```python
from build123d import *

# Parameters (mm, degrees)
SKETCH1_R                                  = 55
SKETCH1_R_2                                = 5
BOSS_EXTRUDE1_DEPTH                        = 11
SKETCH2_R                                  = 7.5
CUT_EXTRUDE1_DEPTH                         = 1
SKETCH3_R                                  = 7
CUT_EXTRUDE2_DEPTH                         = 4
MIRROR1_AT_THE_SECOND_PLANE_COPY_1_SKETC_R = 7.5
MIRROR1_AT_THE_SECOND_PLANE_COPY_1_DEPTH   = 1
MIRROR1_AT_THE_SECOND_PLANE_COPY_2_SKETC_R = 7
MIRROR1_AT_THE_SECOND_PLANE_COPY_2_DEPTH   = 4
FILLET1_R                                  = 200


with BuildPart() as part:
    # Sketch1 → Boss-Extrude1 (new, symmetric)
    with BuildSketch(Plane(origin=(0, 0, 0), x_dir=(0, 0, -1), z_dir=(1, 0, 0))):
        with BuildLine():
            Line((-62.214626272, 32.083333333), (-13.33170563, 126.875))
            ThreePointArc((-13.33170563, 126.875), (0, 135), (13.33170563, 126.875))
            Line((13.33170563, 126.875), (51.962948302, 51.962948302))
            Line((51.962948302, 51.962948302), (126.875, 13.33170563))
            ThreePointArc((126.875, 13.33170563), (135, 0), (126.875, -13.33170563))
            Line((126.875, -13.33170563), (32.083333333, -62.214626272))
            ThreePointArc((32.083333333, -62.214626272), (-49.497474683, -49.497474683), (-62.214626272, 32.083333333))
        make_face()
        Circle(SKETCH1_R, mode=Mode.SUBTRACT)
        with Locations((0, 120)):
            Circle(SKETCH1_R_2, mode=Mode.SUBTRACT)
        with Locations(Location((120, 0, 0), (0, 0, 180))):
            Circle(SKETCH1_R_2, mode=Mode.SUBTRACT)
    extrude(amount=BOSS_EXTRUDE1_DEPTH, both=True)

    # Sketch2 → Cut-Extrude1 (cut)
    with BuildSketch(Plane(origin=(11, 0, 0), x_dir=(0, 0, -1), z_dir=(1, 0, 0))):
        with Locations((0, 120)):
            Circle(SKETCH2_R)
    cut_extrude1 = extrude(amount=-CUT_EXTRUDE1_DEPTH, mode=Mode.SUBTRACT)

    # Sketch3 → Cut-Extrude2 (cut)
    with BuildSketch(Plane(origin=(10, 0, 0), x_dir=(0, 0, -1), z_dir=(1, 0, 0))):
        with Locations((0, 120)):
            Circle(SKETCH3_R)
    cut_extrude2 = extrude(amount=-CUT_EXTRUDE2_DEPTH, mode=Mode.SUBTRACT)

    # Mirror1: Cut-Extrude1, Cut-Extrude2 across plane
    add(cut_extrude1.mirror(Plane(origin=(0, 0, 0), x_dir=(0, -0.7071067811865464, 0.7071067811865487), z_dir=(0, -0.7071067811865487, -0.7071067811865464))), mode=Mode.SUBTRACT)
    add(cut_extrude2.mirror(Plane(origin=(0, 0, 0), x_dir=(0, -0.7071067811865464, 0.7071067811865487), z_dir=(0, -0.7071067811865487, -0.7071067811865464))), mode=Mode.SUBTRACT)

    # Mirror1 at the second plane: Cut-Extrude1, Cut-Extrude2 across plane
    add(cut_extrude1.mirror(Plane(origin=(0, 0, 0), x_dir=(0, 0, 1), z_dir=(1, 0, 0))), mode=Mode.SUBTRACT)
    add(cut_extrude2.mirror(Plane(origin=(0, 0, 0), x_dir=(0, 0, 1), z_dir=(1, 0, 0))), mode=Mode.SUBTRACT)

    # Mirror1 at the second plane copy 1 sketc → Mirror1 at the second plane copy 1 (cut)
    with BuildSketch(Plane(origin=(-11, 0, 0), x_dir=(0, 1, 0), z_dir=(-1, 0, 0))):
        with Locations((0, 120)):
            Circle(MIRROR1_AT_THE_SECOND_PLANE_COPY_1_SKETC_R)
    extrude(amount=-MIRROR1_AT_THE_SECOND_PLANE_COPY_1_DEPTH, mode=Mode.SUBTRACT)

    # Mirror1 at the second plane copy 2 sketc → Mirror1 at the second plane copy 2 (cut)
    with BuildSketch(Plane(origin=(-10, 0, 0), x_dir=(0, 1, 0), z_dir=(-1, 0, 0))):
        with Locations((0, 120)):
            Circle(MIRROR1_AT_THE_SECOND_PLANE_COPY_2_SKETC_R)
    extrude(amount=-MIRROR1_AT_THE_SECOND_PLANE_COPY_2_DEPTH, mode=Mode.SUBTRACT)

    # Fillet1
    fillet1_edges = [part.edges().sort_by_distance(p)[0] for p in [
        (0, 51.962948302, -51.962948302),
    ]]
    fillet(fillet1_edges, radius=FILLET1_R)


solid = part.part
```
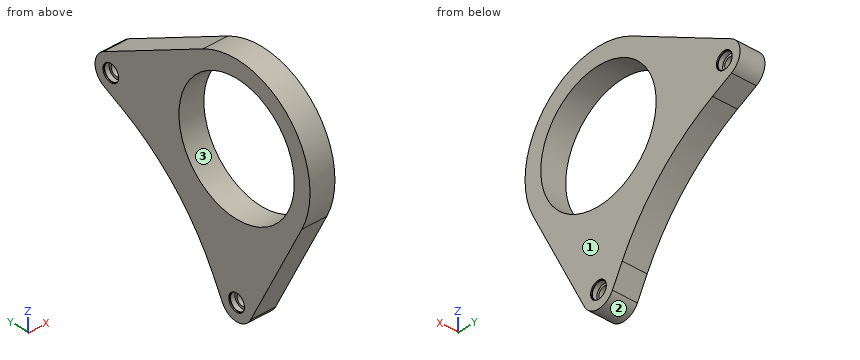
Read the model definition and answer for the solid it produces. Units are mm, in the model's axes. Face numbers are marked on the shaded views. Coordinates: 2 decimals unless noted, no trailing zeros. Loops run counter-clockwise (first coordinate to the right, second up) from the corner with the lowest first, then second, coordinate; pieces in that order, holes last.
(1) The part is cut by section A-A (y = 0). Determine the outline of the cut face in (x, z).
Solution:
outline: (-11, -135) - (11, -135) - (11, -127.5) - (10, -127.5) - (10, -127) - (6, -127) - (6, -125) - (-6, -125) - (-6, -127) - (-10, -127) - (-10, -127.5) - (-11, -127.5) - close; (-11, -112.5) - (-10, -112.5) - (-10, -113) - (-6, -113) - (-6, -115) - (6, -115) - (6, -113) - (10, -113) - (10, -112.5) - (11, -112.5) - (11, -55) - (-11, -55) - close; (-11, 55) - (11, 55) - (11, 70) - (-11, 70) - close
(2) The part is cut by section D-D (z = 33). Determine the outline of the cut face in (x, y).
Solution:
outline: (-11, -61.73) - (11, -61.73) - (11, -44) - (-11, -44) - close; (-11, 44) - (11, 44) - (11, 88.74) - (-11, 88.74) - close
(3) The part is cut by section C-C (x = 3). Determine the outline of the cut face in (y, z) (3 decimals), and give its area (3 significant figures).
Solution:
outline: (-62.215, -32.083) - (-13.332, -126.875) arc R15 ccw to (13.332, -126.875) - (22.672, -108.762) arc R200 cw to (108.762, -22.672) - (126.875, -13.332) arc R15 ccw to (126.875, 13.332) - (32.083, 62.215) arc R70 ccw to start; hole circle Ø110 at (0, 0); hole circle Ø10 at (0, -120); hole circle Ø10 at (120, 0)
area: 14,000 mm2
(4) Consider line 1 along Y through (x, z) = (-1, 0); line 2 along Y through (x, z) = (10.5, 0); line 3 along Z through (x, y) = (2, -3). Determine where each line is inside the solid, lowest interval first.
Solution:
line 1: y = -70 to -55, 55 to 115, 125 to 135
line 2: y = -70 to -55, 55 to 112.5, 127.5 to 135
line 3: z = -134.7 to -124, -116 to -54.92, 54.92 to 69.94
(5) The mould has two halves that part along Y. Classify the marked faces 1, 2 and 3: released by +Y, released by -Y, zero draft, split by the parting line, or undercut.
Solution:
face 1: zero draft
face 2: split by the parting line
face 3: undercut
(6) Flat-ended cylindrical pins translate along their axes: pin 1 Ø5 at (x, z) = (-8, -82) entering from -Y; pin 2 Ø13 at (y, z) = (0, -120) entering from +X; pin 3 Ø13.5 at (y, z) = (120, 0) entering from -X. Find the tip coordinate at first contact, or state that the pin passes through.
Solution:
pin 1: stops at y = -37.76
pin 2: stops at x = 6
pin 3: stops at x = -6
(7) The part is cut by section B-B (z = 0). Determine the outline of the cut face in (x, y).
Solution:
outline: (-11, -70) - (11, -70) - (11, -55) - (-11, -55) - close; (-11, 55) - (11, 55) - (11, 112.5) - (10, 112.5) - (10, 113) - (6, 113) - (6, 115) - (-6, 115) - (-6, 113) - (-10, 113) - (-10, 112.5) - (-11, 112.5) - close; (-11, 127.5) - (-10, 127.5) - (-10, 127) - (-6, 127) - (-6, 125) - (6, 125) - (6, 127) - (10, 127) - (10, 127.5) - (11, 127.5) - (11, 135) - (-11, 135) - close
